Autodesk Inventor part; units mm, degrees
ref_plane "YZ Plane" through (0, 0, 0) normal (1, 0, 0) x (0, 1, 0)
ref_plane "XZ Plane" through (0, 0, 0) normal (0, 1, 0) x (-1, 0, 0)
ref_plane "XY Plane" through (0, 0, 0) normal (0, 0, 1) x (1, 0, 0)
sketch "Sketch1" plane through (0, 0, 0) normal (0, 0, 1) x (1, 0, 0)
  line L0 (-78.24, 3.5741) -> (4.16, 3.5741)
  line L1 (4.16, 3.5741) -> (4.16, -28.8259)
  line L2 (4.16, -28.8259) -> (-78.24, -28.8259)
  line L3 (-78.24, -28.8259) -> (-78.24, 3.5741)
  line L4 (-77.04, 2.3741) -> (2.96, 2.3741)
  line L5 (2.96, 2.3741) -> (2.96, -27.6259)
  line L6 (2.96, -27.6259) -> (-77.04, -27.6259)
  line L7 (-77.04, -27.6259) -> (-77.04, 2.3741)
  point P0 (0, 0)
  dimension "d0" = 32.4
  dimension "d1" = 82.4
  dimension "d2" = 1.2
  dimension "d3" = 1.2
  dimension "d4" = 1.2
  dimension "d5" = 1.2
extrude "Extrusion1" add sketch "Sketch1" along normal blind 25
sketch "Sketch2" plane through (0, 0, 25) normal (0, 0, 1) x (1, 0, 0)
  line L0 (-78.24, 3.5741) -> (4.16, 3.5741)
  line L1 (4.16, 3.5741) -> (4.16, -28.8259)
  line L2 (4.16, -28.8259) -> (-78.24, -28.8259)
  line L3 (-78.24, -28.8259) -> (-78.24, 3.5741)
  point P0 (0, 0)
extrude "Extrusion2" add sketch "Sketch2" along normal blind 1.2
sketch "Sketch3" plane through (-78.24, -28.8259, 0) normal (-1, 0, 0) x (0, 0, 1)
  line L0 (25, 1.2) -> (25, 31.2)
  line L1 (25, 12.45) -> (22, 12.45)
  line L2 (22, 12.45) -> (22, 19.95)
  line L3 (22, 19.95) -> (25, 19.95)
  line L4 (25, 19.95) -> (25, 12.45)
  line L5 (0, 1.2) -> (25, 1.2)
  line L6 (0, 31.2) -> (25, 31.2)
  point P0 (0, 28.8259)
  dimension "d10" = 7.5
  dimension "d11" = 3
  dimension "d12" = 11.25
  dimension "d13" = 11.25
extrude "Extrusion3" cut sketch "Sketch3" against normal blind 1.2
sketch "Sketch4" plane through (0, 0, 25) normal (0, 0, -1) x (-1, 0, 0)
  point P0 (0, 0)
sketch "Sketch5" plane through (0, 0, 25) normal (0, 0, -1) x (-1, 0, 0)
  line L0 (18.04, -7.6259) -> (19.04, -7.6259)
  line L1 (19.04, -7.6259) -> (19.04, -17.6259)
  line L2 (19.04, -17.6259) -> (18.04, -17.6259)
  line L3 (18.04, -17.6259) -> (18.04, -7.6259)
  line L4 (-2.96, 2.3741) -> (77.04, 2.3741)
  line L5 (77.04, -27.6259) -> (-2.96, -27.6259)
  line L6 (77.04, 2.3741) -> (77.04, -27.6259)
  point P0 (0, 0)
  dimension "d16" = 1
  dimension "d17" = 10
  dimension "d18" = 10
  dimension "d19" = 10
  dimension "d20" = 58
extrude "Extrusion4" add sketch "Sketch5" along normal blind 1.5
chamfer "Chamfer1" distance 1.5 angle 45 2 edges at (-18.54, -17.6259, 23.5) (-18.54, -7.6259, 23.5)
chamfer "Chamfer2" distance 1.5 angle 45 1 edges at (-18.04, -12.6259, 25)
sketch "Sketch6" plane through (-78.24, -28.8259, 0) normal (0, -1, 0) x (1, 0, 0)
  circle A0 centre (3.7, 12.5) radius 2.5
  line L0 (1.2, 0) -> (1.2, 25)
  point P0 (78.24, 0)
  dimension "d29" = 5
  dimension "d30" = 2.5
extrude "Extrusion5" cut sketch "Sketch6" against normal blind 40
sketch "Sketch7" plane through (4.16, -28.8259, 0) normal (1, 0, 0) x (0, 0, -1)
  line L0 (0, 31.2) -> (-25, 31.2)
  line L1 (0, 32.4) -> (0, 0)
  circle A0 centre (-8, 26.2) radius 1.5
  circle A1 centre (-8, 21.2) radius 1.5
  circle A2 centre (-8, 16.2) radius 1.5
  circle A3 centre (-8, 11.2) radius 1.5
  circle A4 centre (-8, 6.2) radius 1.5
  line L2 (0, 1.2) -> (-25, 1.2)
  point P0 (0, 28.8259)
  point P1 (-8, 31.2)
  dimension "d33" = 8
  dimension "d34" = 3
  dimension "d35" = 3
  dimension "d36" = 3
  dimension "d37" = 3
  dimension "d38" = 3
  dimension "d39" = 5
  dimension "d40" = 5
  dimension "d41" = 5
  dimension "d42" = 5
  dimension "d43" = 5
  dimension "d44" = 5
extrude "Extrusion6" cut sketch "Sketch7" against normal blind 3
sketch "Sketch8" plane through (0, 0, 0) normal (0, 0, -1) x (-1, 0, 0)
  line L0 (78.24, -28.8259) -> (-4.16, -28.8259)
  line L1 (-4.16, -28.8259) -> (-4.16, -30.0259)
  line L2 (-4.16, -30.0259) -> (78.24, -30.0259)
  line L3 (78.24, -30.0259) -> (78.24, -28.8259)
  line L4 (78.24, 3.5741) -> (-4.16, 3.5741)
  line L5 (-4.16, 3.5741) -> (-4.16, 4.7741)
  line L6 (-4.16, 4.7741) -> (78.24, 4.7741)
  line L7 (78.24, 4.7741) -> (78.24, 3.5741)
  line L8 (-4.16, 3.5741) -> (-4.16, -28.8259)
  point P0 (0, 0)
  dimension "d47" = 1.2
  dimension "d48" = 1.2
extrude "Extrusion7" add sketch "Sketch8" against normal blind 26.2
sketch "Sketch9" plane through (0, 0, 0) normal (0, 0, -1) x (-1, 0, 0)
  line L0 (-2.96, -27.6259) -> (77.04, -27.6259)
  line L1 (77.04, -27.6259) -> (77.04, -28.8259)
  line L2 (77.04, -28.8259) -> (-2.96, -28.8259)
  line L3 (-2.96, -28.8259) -> (-2.96, -27.6259)
  line L4 (77.04, 2.3741) -> (-2.96, 2.3741)
  line L5 (-2.96, 2.3741) -> (-2.96, 3.5741)
  line L6 (-2.96, 3.5741) -> (77.04, 3.5741)
  line L7 (77.04, 3.5741) -> (77.04, 2.3741)
  line L8 (-2.96, 2.3741) -> (77.04, 2.3741)
  line L9 (77.04, 2.3741) -> (77.04, -27.6259)
  point P0 (0, 0)
  dimension "d51" = 1.2
  dimension "d52" = 1.2
extrude "Extrusion8" cut sketch "Sketch9" against normal blind 25
sketch "Sketch10" plane through (-78.24, -30.0259, 0) normal (-1, 0, 0) x (0, 0, 1)
  line L0 (25, 21.15) -> (25, 33.6)
  line L1 (22, 13.45) -> (25, 13.45)
  line L2 (25, 13.45) -> (25, 21.35)
  line L3 (25, 21.35) -> (22, 21.35)
  line L4 (22, 21.35) -> (22, 13.45)
  line L5 (25, 13.65) -> (22, 13.65)
  line L6 (22, 21.15) -> (25, 21.15)
  line L7 (22, 13.65) -> (22, 21.15)
  point P0 (0, 30.0259)
  dimension "d55" = 0.2
  dimension "d56" = 0.2
extrude "Extrusion9" cut sketch "Sketch10" against normal blind 2
sketch "Sketch11" plane through (0, 0, 25) normal (0, 0, -1) x (-1, 0, 0)
  point P0 (0, 0)
properties part number "Case Botom v2"
Geometry: final body of the model. Coordinates: model frame, mm. A direction names the side the tool comes from. Coordinates: 2 decimals unless noted, no trailing zeros. Order: outer loops, then holes, each group sorted by start corner. A loop starts at its lowest first (then second) coordinate and runs counter-clockwise, first axis right, second up. Notation, with made-up numbers: M 52.25,-25.5 L 57.25,-25.5 A19 cw 57.25,-10.5 Z; hole C 66.5,-33 d7. An arc over 180 degrees is marked long. Answer as CSV lines item,"result".
Q1. Draft query along Z for faces 4 (the flat face through (-37, 4, 0)), 5 (the flat face through (-36, 4.774, 13)), 6 (the cylindrical face through (3.6, -12.6, 9.5)). Return one class per face: pulls with the +Z half, pulls with the -Z half, needs draft (parallel to the pull), parting line crosses it, or undercut.
Answers:
face 4,"pulls with the -Z half"
face 5,"needs draft"
face 6,"undercut"
Q2. Section C-C on z = 8. Return the cut outline in (x, y).
Answers:
outline,"M -78.24,-30.03 L 4.16,-30.03 L 4.16,-24.13 L 2.96,-24.13 L 2.96,-28.83 L -77.04,-28.83 L -77.04,3.57 L 2.96,3.57 L 2.96,-1.13 L 4.16,-1.13 L 4.16,4.77 L -78.24,4.77 Z; M 2.96,-21.13 L 4.16,-21.13 L 4.16,-19.13 L 2.96,-19.13 Z; M 2.96,-16.13 L 4.16,-16.13 L 4.16,-14.13 L 2.96,-14.13 Z; M 2.96,-11.13 L 4.16,-11.13 L 4.16,-9.13 L 2.96,-9.13 Z; M 2.96,-6.13 L 4.16,-6.13 L 4.16,-4.13 L 2.96,-4.13 Z"
Q3. Section D-D on y = -5. Return the cut outline in (x, z).
Answers:
outline,"M -78.24,0 L -77.04,0 L -77.04,25 L 2.96,25 L 2.96,0 L 4.16,0 L 4.16,26.2 L -78.24,26.2 Z"
Q4. Section B-B on x = -25. Return the cut outline in (y, z).
Answers:
outline,"M -30.03,0 L -28.83,0 L -28.83,25 L 3.57,25 L 3.57,0 L 4.77,0 L 4.77,26.2 L -30.03,26.2 Z"
Q5. Line query: probe 1 along Y at (x, z) = (3.6, 8); probe 2 along X at (y, z) = (-15, 10.75); probe 3 along Y at (x, z) = (-1, 2.25). Output: solid intervals per line, ascending. Write a range as [from, to].
Answers:
probe 1,"y = [-30.03, -24.13], [-21.13, -19.13], [-16.13, -14.13], [-11.13, -9.13], [-6.13, -4.13], [-1.13, 4.77]"
probe 2,"x = [-78.24, -77.04], [2.96, 4.16]"
probe 3,"y = [-30.03, -28.83], [3.57, 4.77]"
Q6. Set-up query: faces 1 (the cylindrical face through (3.568, -1.612, 9.106)), 2 (the flat face through (-78.24, -13, 13)), 3 (the flat face through (-77.04, -13, 12)). Return all of +Z, -Z, +X, -X, +Y, -Y with unobstructed straight access to the full face (end or side cutting, diameter ignored); none if empty.
Answers:
face 1,"+X"
face 2,"+Z, -Z, -X, +Y, -Y"
face 3,"-Z"
Q7. First-contact query: P1, Ø6, axis at x = -37, y = -17.5, coming from the -Z side; P2, Ø2.5, axis at y = -7.63, z = 8, coming from the +X side; P3, Ø0.5, axis at x = -18.5, y = -11, coming from the -Z side; P4, Ø3.5, axis at y = -12.63, z = 8, coming from the +X side. Flat tips, straight axial feed; report the tip coordinate or a pass-through.
Answers:
P1,"stops at z = 25"
P2,"stops at x = -77.04"
P3,"stops at z = 23.5"
P4,"stops at x = 4.16"
Q8. Section A-A on z = 20. Return the cut outline in (x, y), and give its area (3 significant figures).
Answers:
outline,"M -78.24,-30.03 L 4.16,-30.03 L 4.16,4.77 L -78.24,4.77 Z; hole M -77.04,-28.83 L 2.96,-28.83 L 2.96,3.57 L -77.04,3.57 Z"
area,"276 mm^2"
